Build history of the part. All positions in model axes, mm. Give positions to 0.01 mm unless a question says otherwise; leave off trailing zeros. Order: outer loops, then holes, each group sorted by start corner. A loop starts at its lowest first (then second) coordinate and runs counter-clockwise, first axis right, second up. Notation, with made-up numbers: (55.5, 72) -> (111.5, 72) arc R18 cw to (111.5, 97) -> close; hole circle Ø11 at (75.25, -17.5). An arc over 180 degrees is marked (long way). Write item = value, one per line. Start each with the question number.
from build123d import *

# Parameters (mm, degrees)
F0_R     = 2
F1_DEPTH = 3.2
F4_R     = 0.1
F5_R     = 0.1


with BuildPart() as f1:
    # F0 (on Top) → F1 (new body)
    with BuildSketch(Plane.XY):
        Polygon((-3.5, -2.020726), (0, -4.041452), (3.5, -2.020726), (3.5, 2.020726), (0, 4.041452), (-3.5, 2.020726), align=None)
        Circle(F0_R, mode=Mode.SUBTRACT)
    extrude(amount=F1_DEPTH)

    # F2 (on Front) → F3 (revolve, cut)
    with BuildSketch(Plane.XZ):
        Polygon((4.614809, 3.2), (3.5, 3.2), (4.614809, 2.556365), align=None)
        Polygon((4.614809, 2.556365), (3.5, 3.2), (2.75, 3.2), (4.614809, 2.123352), align=None)
        Polygon((5.364809, 3.2), (4.614809, 3.2), (4.614809, 2.556365), (5.364809, 2.123352), align=None)
        Polygon((4.614809, 0.643635), (3.5, 0), (4.614809, 0), align=None)
        Polygon((2.75, 0), (3.5, 0), (4.614809, 0.643635), (4.614809, 1.076648), align=None)
        Polygon((4.614809, 0.643635), (4.614809, 0), (5.364809, 0), (5.364809, 1.076648), align=None)
    revolve(axis=Axis((0, 0, 1.6), (0, 0, 1)), mode=Mode.SUBTRACT)

    # F4
    f4_edges = [f1.edges().sort_by_distance(p)[0] for p in [
        (-2, 0, 3.2),
    ]]
    fillet(f4_edges, radius=F4_R)

    # F5
    f5_edges = [f1.edges().sort_by_distance(p)[0] for p in [
        (-2, 0, 0),
    ]]
    fillet(f5_edges, radius=F5_R)


solid = f1.part
(1) Cut at C-C, the plane z = 2.65. Give the cut face in (x, y).
(2) Wall check: line 1 (X direction, y = -0.25, z = 2.05); line 2 (Y direction, x = -1.25, z = 2.9); line 3 (X direction, y = -1, z = 0.6). Give the ranges that are in metal, low to high. Write a range as [from, to].
(3) Cut at A-A, the plane y = 0. Give the cut face in (x, z), plus the area to 3 significant figures.
(4) Cut at B-B, the plane z = 1.75. Give the cut face in (x, y).
(5) Flat gauge pin, fed straight in: P1, Ø1.5, axis at x = -2, z = 2.5, coming from the +Y side. Where does the tip first touch, or does it go through?
Results:
q1.outline = (-3.5, -1.21) arc R3.7 ccw to (-2.8, -2.43) -> (-0.7, -3.64) arc R3.7 ccw to (0.7, -3.64) -> (2.8, -2.43) arc R3.7 ccw to (3.5, -1.21) -> (3.5, 1.21) arc R3.7 ccw to (2.8, 2.43) -> (0.7, 3.64) arc R3.7 ccw to (-0.7, 3.64) -> (-2.8, 2.43) arc R3.7 ccw to (-3.5, 1.21) -> close; hole circle Ø4 at (0, 0)
q2.line_1 = [-3.5, -1.98], [1.98, 3.5]
q2.line_2 = [-3.02, -1.56], [1.56, 3.02]
q2.line_3 = [-3.5, -1.73], [1.73, 3.5]
q3.outline = (-3.5, 0.43) -> (-2.75, 0) -> (-2.1, 0) arc R0.1 ccw to (-2, 0.1) -> (-2, 3.1) arc R0.1 ccw to (-2.1, 3.2) -> (-2.75, 3.2) -> (-3.5, 2.77) -> close; (2, 0.1) arc R0.1 ccw to (2.1, 0) -> (2.75, 0) -> (3.5, 0.43) -> (3.5, 2.77) -> (2.75, 3.2) -> (2.1, 3.2) arc R0.1 ccw to (2, 3.1) -> close
q3.area = 8.94 mm2
q4.outline = (-3.5, -2.02) -> (0, -4.04) -> (3.5, -2.02) -> (3.5, 2.02) -> (0, 4.04) -> (-3.5, 2.02) -> close; hole circle Ø4 at (0, 0)
q5.P1 = 3.32
